```python
from build123d import *

# Parameters (mm, degrees)
FILLET1_R     = 2
CHAMFER1_SIZE = 0.2


with BuildPart() as part:
    # Sketch1 → Revolve1 (revolve)
    with BuildSketch(Plane.XY, mode=Mode.PRIVATE) as revolve1_sk:
        Polygon((0, 46.355), (0, 27.305), (6.35, 27.305), (6.35, 26), (53.98, 26), (53.98, 26.8), (64.14, 26.8), (64.14, 46.1), (53.98, 46.1), (53.98, 47.37), (6.35, 47.37), (6.35, 46.355), align=None)
    revolve(revolve1_sk.sketch.rotate(Axis((0, 0, 0), (1, 0, 0)), 90), axis=Axis((0, 0, 0), (1, 0, 0)))

    # Fillet1
    fillet1_edges = [part.edges().sort_by_distance(p)[0] for p in [
        (64.14, 0, -46.1),
        (64.14, 0, -26.8),
        (0, 0, -27.305),
        (0, 0, -46.355),
    ]]
    fillet(fillet1_edges, radius=FILLET1_R)

    # Chamfer1
    chamfer1_edges = [part.edges().sort_by_distance(p)[0] for p in [
        (53.98, 0, -47.37),
        (6.35, 0, -47.37),
    ]]
    chamfer(chamfer1_edges, length=CHAMFER1_SIZE)


solid = part.part
```
CAD build for the part. Positions are in the model's coordinates, mm. A direction names the side the tool comes from. Coordinates: 2 decimals unless noted, no trailing zeros. Write each loop counter-clockwise with the first axis right and the second up, starting at its lowest first coordinate (ties: lowest second). Pieces come first, ordered by that corner, then holes. Notation, with made-up numbers: (52, -31.5) -> (57, -31.5) arc R9 cw to (57, -26.5) -> close; hole circle Ø5 at (-39, -31.75). An arc over 180 degrees is marked (long way). Use CSV: the item, a comma, the result in double quotes. Start each with the question number.
Item 1: Band-saw the part on A-A, the plane x = 24.5. Write the cut outline in (y, z).
Item 2: Drop flat-ended pins along their axis: P1, Ø4, axis at x = 46.5, z = 21, coming from the +Y side; P2, Ø12, axis at x = 34, z = 4, coming from the -Y side; P3, Ø1, axis at x = 29, y = -21, coming from the +Z side. Give the stop position or say it passes through.
Item 3: Band-saw the part on B-B, the plane x = 60.5. Write the cut outline in (y, z).
Item 4: Tool access for faces 1 (the flat face through (6.35, 22.1, 14)), 2 (the flat face through (0, 29, 9)), 3 (the flat face through (53.98, -4, 26)): list every direction of +Z, -Z, +X, -X, +Y, -Y with a clear straight run to the whole face (end or side of a thin tool).
Item 5: Two-plate mould, pull along Y, no slides. Class faces 4 (the flat face through (6.35, 31, 35)), 5 (the cylindrical face through (30.498, 15.821, -20.633)), 6 (the cylindrical face through (58, -13.85, 43.97)): +Y half, -Y half, draft (parallel to the pull), parting line (faces both ways), or undercut.
Item 6: Wall check: probe 1 along Y at (x, z) = (4, 0) (3 decimals); probe 2 along Y at (x, z) = (44, 0); probe 3 along Y at (x, z) = (28, 38). Give the ranges that are in metal, low to high.
Response values:
1,outline,"circle Ø94.74 at (0, 0); hole circle Ø52 at (0, 0)"
2,P1,"stops at y = 43.39"
2,P2,"stops at y = -47.37"
2,P3,"stops at z = 42.7"
3,outline,"circle Ø92.2 at (0, 0); hole circle Ø53.6 at (0, 0)"
4,face 1,"-X"
4,face 2,"+Z, -Z, -X, +Y, -Y"
4,face 3,"+X"
5,face 4,"draft"
5,face 5,"undercut"
5,face 6,"parting line"
6,probe 1,"y = -46.355 to -27.305, 27.305 to 46.355"
6,probe 2,"y = -47.37 to -26, 26 to 47.37"
6,probe 3,"y = -28.28 to 28.28"
